Can you work these out from the model? Positions are in its coordinate system, mm. Face numbers are marked on the shaded views. Coordinates: 2 decimals unless noted, no trailing zeros. Write each loop counter-clockwise with the first axis right and the second up, starting at its lowest first coordinate (ties: lowest second). Pieces come first, ordered by that corner, then holes. Notation, with made-up numbers: (2, 61.5) -> (45, 61.5) arc R33 cw to (45, 98.5) -> close; hole circle Ø5 at (-10.5, -26). An arc over 180 degrees is marked (long way). Use one line per item in the form item = value.
```python
from build123d import *

# Parameters (mm, degrees)
SKETCH1_R           = 4
SKETCH1_R_2         = 1.5
BOSS_EXTRUDE1_DEPTH = 2
CHAMFER1_SIZE       = 1.9
CHAMFER2_SIZE       = 0.25


with BuildPart() as part:
    # Sketch1 → Boss-Extrude1 (new body)
    with BuildSketch(Plane(origin=(0, 0, 0), x_dir=(0, 0, -1), z_dir=(1, 0, 0))):
        Circle(SKETCH1_R)
        Circle(SKETCH1_R_2, mode=Mode.SUBTRACT)
    extrude(amount=BOSS_EXTRUDE1_DEPTH)

    # Chamfer1
    chamfer1_edges = [part.edges().sort_by_distance(p)[0] for p in [
        (2, 0, 1.5),
    ]]
    chamfer(chamfer1_edges, length=CHAMFER1_SIZE)

    # Chamfer2
    chamfer2_edges = [part.edges().sort_by_distance(p)[0] for p in [
        (0, 0, 4),
        (2, 0, 4),
    ]]
    chamfer(chamfer2_edges, length=CHAMFER2_SIZE)


solid = part.part
```
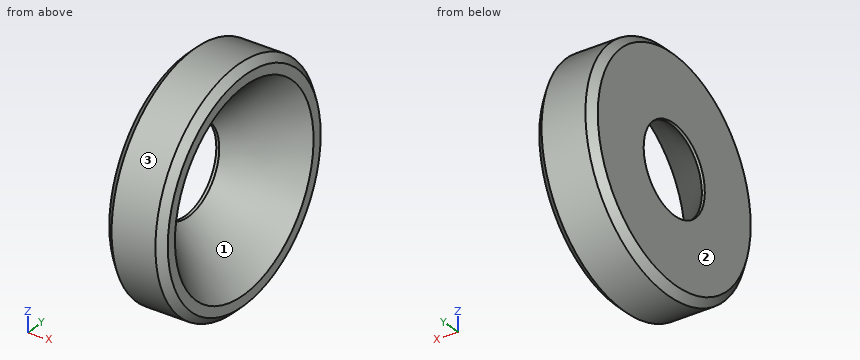
Q1. If I drill on line 1 (Z direction, x = 0.8, y = 0.25); line 2 (Y direction, x = 0.15, z = 0); line 3 (Z direction, x = 1.3, y = -1.75), over which ranges is the centre line in solid material (lowest first)? Write a range as from..to.
Return value:
line_1 = -3.99..-2.19, 2.19..3.99
line_2 = -3.9..-1.55, 1.55..3.9
line_3 = -3.6..-2.06, 2.06..3.6
Q2. Suppose I cut it at A-A (y = 0). Write out the boundary of the cut face in (x, z).
Return value:
outline = (0, -3.75) -> (0.25, -4) -> (1.75, -4) -> (2, -3.75) -> (2, -3.4) -> (0.1, -1.5) -> (0, -1.5) -> close; (0, 1.5) -> (0.1, 1.5) -> (2, 3.4) -> (2, 3.75) -> (1.75, 4) -> (0.25, 4) -> (0, 3.75) -> close
Q3. Will these pins go through, and if not, where does the flat tip stop? pin 1 (4 mm diameter, centred on y = 0, z = 0, fed in from +X); pin 2 (1 mm diameter, centred on x = 1, z = -1.5, fed in from +Y).
Return value:
pin_1 = 0.6
pin_2 = 3.87
Q4. Suppose I cut it at C-C (x = 0.85). Write out the boundary of the cut face in (y, z), then the cut area to 3 significant figures.
Return value:
outline = circle Ø8 at (0, 0); hole circle Ø4.5 at (0, 0)
area = 34.4 mm2
Q5. Thinking about a two-plate mould opening in Y: for the marked faces 1, 2 and 3, which applies, released by +Y, released by -Y, zero draft, split by the parting line, or undercut?
Return value:
face_1 = undercut
face_2 = zero draft
face_3 = split by the parting line
